```python
from build123d import *

# Parameters (mm, degrees)
F1_DEPTH = 15.24
F2_W     = 12.446
F2_H     = 10.4394
F3_DEPTH = 9.017
F5_DEPTH = 10.16


with BuildPart() as f1:
    # F0 (on Top) → F1 (new body)
    with BuildSketch(Plane.XY):
        with BuildLine():
            Line((3.388283, 5.2197), (-3.388283, 5.2197))
            ThreePointArc((-3.388283, 5.2197), (-6.223, 0), (-3.388283, -5.2197))
            Line((-3.388283, -5.2197), (3.388283, -5.2197))
            ThreePointArc((3.388283, -5.2197), (6.223, 0), (3.388283, 5.2197))
        make_face()
    extrude(amount=F1_DEPTH)

    # F2 (on face) → F3 (join)
    with BuildSketch(Plane.XY.offset(15.24)):
        Rectangle(F2_W, F2_H)
    extrude(amount=F3_DEPTH)

    # F4 (on face) → F5 (join)
    with BuildSketch(Plane.XY.offset(24.257)):
        with BuildLine():
            Line((-1.15814, -0.9906), (1.15814, -0.9906))
            ThreePointArc((1.15814, -0.9906), (0, 1.524), (-1.15814, -0.9906))
        make_face()
    extrude(amount=F5_DEPTH)


solid = f1.part
```
Source: CAD feature listing. Evaluate the final solid. Frame: model axes, mm. A direction names the side the tool comes from. Coordinates: 2 decimals unless noted, no trailing zeros. Write each loop counter-clockwise with the first axis right and the second up, starting at its lowest first coordinate (ties: lowest second). Pieces come first, ordered by that corner, then holes. Notation, with made-up numbers: M 64.5,79 L 80.5,79 A25 ccw 80.5,100 Z; hole C 25.5,74.5 d10. An arc over 180 degrees is marked long. Answer as a JSON object with one key per item and string values.
1. Cut plane A-A on x = 0. Output: boundary loops of the cut face in (y, z).
Evaluation:
{"outline": "M -5.22,0 L 5.22,0 L 5.22,24.26 L 1.52,24.26 L 1.52,34.42 L -0.99,34.42 L -0.99,24.26 L -5.22,24.26 Z"}
2. Contact query for flat-ended pins moving along their axis: P1, Ø4, axis at x = 2, y = -2, coming from the -Z side; P2, Ø1.5, axis at x = -4, z = 29, coming from the +Y side; P3, Ø3, axis at x = -0.5, z = 29.5, coming from the +Y side; P4, Ø6, axis at x = 3.5, y = 4, coming from the +Z side. Output: stop coordinate, or through.
Evaluation:
{"P1": "z = 0", "P2": "through", "P3": "y = 1.52", "P4": "z = 24.26"}
3. Cut plane C-C on z = 31.5. Output: boundary loops of the cut face in (x, y).
Evaluation:
{"outline": "M -1.16,-0.99 L 1.16,-0.99 A1.52 ccw long Z"}
4. Ray query, L1, parallel to Z at x = -3, y = -3.5; L2, parallel to Z at x = 5.75, y = -4; L3, parallel to X at y = 1.75, z = 4. Return the intervals inside material, ascending.
Evaluation:
{"L1": "0 to 24.26", "L2": "15.24 to 24.26", "L3": "-5.97 to 5.97"}
5. Access query for faces 1 (the flat face through (0, -0.991, 29)), 2 (the cylindrical face through (6.222, -0.087, 7.513)), 3 (the flat face through (-5, -4, 15.24)), 4 (the cylindrical face through (-6.222, 0.087, 7.513)), 5 (the flat face through (-5, 4, 15.24)). Directions: +Z, -Z, +X, -X, +Y, -Y. A direction counts if a zero-diameter tool reaches every point of the face in a straight line with its end or side. Return the directions, or none.
Evaluation:
{"face 1": "+Z, +X, -X, -Y", "face 2": "-Z, +X", "face 3": "-Z, -X, -Y", "face 4": "-Z, -X", "face 5": "-Z, -X, +Y"}
6. Cut plane D-D on x = -2.5. Output: boundary loops of the cut face in (y, z), plus the area to 3 significant figures.
Evaluation:
{"outline": "M -5.22,0 L 5.22,0 L 5.22,24.26 L -5.22,24.26 Z", "area": "253 mm^2"}
7. Cut plane B-B on y = -2. Output: boundary loops of the cut face in (x, z), plus the area to 3 significant figures.
Evaluation:
{"outline": "M -6.22,15.24 L -5.89,15.24 L -5.89,0 L 5.89,0 L 5.89,15.24 L 6.22,15.24 L 6.22,24.26 L -6.22,24.26 Z", "area": "292 mm^2"}
